Verification items for the finished model (mm, model axes). A direction names the side the tool comes from. Give positions to 0.01 mm unless a question says otherwise; leave off trailing zeros. Loops run counter-clockwise (first coordinate to the right, second up) from the corner with the lowest first, then second, coordinate; pieces in that order, holes last. Notation, with made-up numbers: (45.5, 21) - (86.5, 21) arc R20 cw to (86.5, 25) - close; hole circle Ø2 at (7, 21). An arc over 180 degrees is marked (long way). Use one line per item in the form item = value.
```python
from build123d import *

# Parameters (mm, degrees)
F0_R          = 18.1930467882
F1_DEPTH      = 30
F2_R          = 15.7731461296
F3_DEPTH      = 25
F5_DEPTH      = 25
F5_DEPTH_BACK = 25
F6_W          = 50.437502563
F6_H          = 30.6197889149
F7_DEPTH      = 25
F7_DEPTH_BACK = 25
F8_DEPTH      = 25
F9_R          = 16.3489622069
F10_DEPTH     = 15.1


with BuildPart() as f1:
    # F0 (on Top) → F1 (new body)
    with BuildSketch(Plane.XY):
        Circle(F0_R)
    extrude(amount=F1_DEPTH)

    # F2 (on face) → F3 (cut)
    with BuildSketch(Plane(origin=(0, 0, 0), x_dir=(1, 0, 0), z_dir=(0, 0, -1))):
        Circle(F2_R)
    extrude(amount=-F3_DEPTH, mode=Mode.SUBTRACT)

    # F4 (on Front) → F5 (cut, two sides)
    with BuildSketch(Plane.XZ) as f5_sk:
        Polygon((0, 24.8274412006), (-18.1874278933, 0), (18.0421601981, 0), align=None)
    extrude(amount=-F5_DEPTH, mode=Mode.SUBTRACT)
    extrude(f5_sk.sketch, amount=F5_DEPTH_BACK, mode=Mode.SUBTRACT)

    # F6 (on Front) → F7 (cut, two sides)
    with BuildSketch(Plane.XZ) as f7_sk:
        with Locations((0, -9.8076611757)):
            Rectangle(F6_W, F6_H)
    extrude(amount=-F7_DEPTH, mode=Mode.SUBTRACT)
    extrude(f7_sk.sketch, amount=F7_DEPTH_BACK, mode=Mode.SUBTRACT)

    # F8 (add): a face of the model
    f8_faces = [f1.faces().sort_by_distance(p)[0] for p in [
        (0, 0, 30),
    ]]
    extrude(f8_faces, amount=F8_DEPTH)

    # F9 (on face) → F10 (cut)
    with BuildSketch(Plane.XY.offset(55)):
        Circle(F9_R)
    extrude(amount=-F10_DEPTH, mode=Mode.SUBTRACT)


solid = f1.part
```
1. Section check A-A, the plane z = 13. Record the cut outline in (x, y).
Result set:
outline = (-8.66, -16) - (-8.66, -13.18) arc R15.77 cw to (-8.66, 13.18) - (-8.66, 16) arc R18.19 ccw to start; (8.6, -16.03) arc R18.19 ccw to (8.6, 16.03) - (8.6, 13.23) arc R15.77 cw to (8.6, -13.23) - close
2. Depth check by flat-ended pin: pin 1 Ø5 at (y, z) = (13.5, 35.5) entering from +X; pin 2 Ø2 at (y, z) = (-7, 45) entering from +X; pin 3 Ø12 at (x, z) = (-12.5, 16.5) entering from -Y. Enter the tip coordinate at first touch or a pass-through.
Result set:
pin_1 = 14.49
pin_2 = 17.18
pin_3 = -16.99
3. Section check C-C, the plane x = 2. Record the cut outline in (y, z).
Result set:
outline = (-18.08, 22.08) - (-15.65, 22.08) - (-15.65, 25) - (15.65, 25) - (15.65, 22.08) - (18.08, 22.08) - (18.08, 55) - (16.23, 55) - (16.23, 39.9) - (-16.23, 39.9) - (-16.23, 55) - (-18.08, 55) - close
4. Tool access check on faces 4 (the flat face through (-16, 0, 5.502)), 5 (the cylindrical face through (7.278, 13.993, 17.281)), 6 (the cylindrical face through (-2.13, 16.21, 47.56)), 7 (the flat face through (-7.57, -14.265, 14.494)), 8 (the flat face through (-15, 7, 55)). Record the directions out of +Z, -Z, +X, -X, +Y, -Y that give a thin tool (end or side, any length) a straight path to the whole face; none if there is none.
Result set:
face_4 = -Z, +X, -X, +Y, -Y
face_5 = -Z
face_6 = +Z
face_7 = -Z, +Y, -Y
face_8 = +Z, +X, -X, +Y, -Y
5. Section check D-D, the plane z = 29.5. Record the cut outline in (x, y).
Result set:
outline = circle Ø36.39 at (0, 0)
6. Draft check along Y on faces 1 (the cylindrical face through (16.806, -6.968, 29.905)), 2 (the flat face through (0, 0, 25)), 3 (the flat face through (16, 0, 5.502)). Enter one of: released by +Y, released by -Y, zero draft, split by the parting line, or undercut.
Result set:
face_1 = split by the parting line
face_2 = undercut
face_3 = zero draft
7. Section check B-B, the plane y = 0. Record the cut outline in (x, z), then the cut area to 3 significant figures.
Result set:
outline = (-18.19, 5.5) - (-15.77, 5.5) - (-15.77, 25) - (15.77, 25) - (15.77, 5.5) - (18.19, 5.5) - (18.19, 55) - (16.35, 55) - (16.35, 39.9) - (-16.35, 39.9) - (-16.35, 55) - (-18.19, 55) - close
area = 692 mm²
8. Scan lines: probe 1 along Y at (x, z) = (0, 50); probe 2 along X at (y, z) = (0, 20.25); probe 3 along Z at (x, y) = (9.5, 6). Record each from-to range of solid material in increasing order.
Result set:
probe_1 = -18.19 to -16.35, 16.35 to 18.19
probe_2 = -18.19 to -15.77, 15.77 to 18.19
probe_3 = 25 to 39.9
